Can you work these out from the model? Positions are in its coordinate system, mm. A direction names the side the tool comes from. Give positions to 0.01 mm unless a question says otherwise; leave off trailing zeros. Write each loop counter-clockwise with the first axis right and the second up, starting at its lowest first coordinate (ties: lowest second). Pieces come first, ordered by that corner, then holes.
1. I'm going to push flat-ended pins straight in: pin 1 (1.9 mm diameter, centred on x = -5.5, z = -10.5, fed in from -Y); pin 2 (1.5 mm diameter, centred on x = -5, z = -13, fed in from +Y); pin 3 (0.6 mm diameter, centred on x = 0.5, z = 0.5, fed in from -Y); pin 4 (1.5 mm diameter, centred on y = 0, z = -13.87, fed in from +X). Where does each tip first touch, or does it pass through?
2. Suppose I cut it at D-D (x = -3.75). Please give me the cut outline in (y, z), and give its area (3 significant figures).
3. If I drill on probe 1 along X at (y, z) = (-2.5, -7.25); probe 2 along Z at (x, y) = (-5.5, 0); probe 3 along Y at (x, z) = (-3.75, -13.75), over which ranges is the centre line in solid material (lowest first)?
4. Suppose I cut it at B-B (z = -8.25). Please give me the cut outline in (x, y), and give its area (3 significant figures).
5. On a 3-axis mill with a long thin cutter (end or side, diameter ignored), from which of +Z, -Z, +X, -X, +Y, -Y can I reach the whole of each face in a straight line? I mean faces 1 (the flat face through (-4, -4, -14.869)), 2 (the flat face through (-4, -5.002, -16)), 3 (the flat face through (1.25, 0, -10)). Say none if no direction works.
6. Thinking about a two-plate mould opening in Y: for faces 4 (the flat face through (4, -4, -14.869)), 5 (the cylindrical face through (-4.419, 0.577, -14.978)), 6 (the flat face through (0, -4, 0)), 7 (the flat face through (0, 4, 0)), which applies, pulls with the +Y half, pulls with the -Y half, needs draft (parallel to the pull), parting line crosses it, or undercut?
7. Suppose I cut it at A-A (y = 0). Please give me the cut outline in (x, z).
8. Suppose I cut it at C-C (z = -13.25). Please give me the cut outline in (x, y), and give its area (3 significant figures).
```python
from build123d import *

# Parameters (mm, degrees)
F0_R     = 1.25
F1_DEPTH = 7.5
F2_R     = 11
F3_DEPTH = 1.25


# Not quite as in the source:
# - a feature of the source that left no trace in its solid (it failed there, or was rolled back) is left out


with BuildPart() as f1:
    # F0 (on Right) → F1 (new body, symmetric)
    with BuildSketch(Plane.YZ):
        with BuildLine():
            Line((4, -1), (4, 1))
            Line((4, 1), (-4, 1))
            Line((-4, 1), (-4, -1))
            Line((-4, -1), (-3.4641016151, -1))
            ThreePointArc((-3.4641016151, -1), (-3.9803488917, -3.39600846), (-3.0021324352, -5.6433313908))
            Line((-3.0021324352, -5.6433313908), (-3.0021324352, -14.8694054575))
            Line((-3.0021324352, -14.8694054575), (-5.0021324352, -14.8694054575))
            Line((-5.0021324352, -14.8694054575), (-5.0021324352, -16.8694054575))
            Line((-5.0021324352, -16.8694054575), (3.9978675648, -16.8694054575))
            Line((3.9978675648, -16.8694054575), (3.9978675648, -14.8694054575))
            Line((3.9978675648, -14.8694054575), (3.9978675648, -3.1305945425))
            Line((3.9978675648, -3.1305945425), (3.9978675648, -2.8694054575))
            ThreePointArc((3.9978675648, -2.8694054575), (3.846285897, -1.901781079), (3.4641016151, -1))
            Line((3.4641016151, -1), (4, -1))
        make_face()
        with Locations((0, -13.8694054575)):
            Circle(F0_R, mode=Mode.SUBTRACT)
        with BuildLine():
            ThreePointArc((3.9978675648, -3.1305945425), (4, -3), (3.9978675648, -2.8694054575))
            Line((3.9978675648, -2.8694054575), (3.9978675648, -3.1305945425))
        make_face()
    extrude(amount=F1_DEPTH, both=True)

    # F2 (on Right) → F3 (cut, symmetric)
    with BuildSketch(Plane.YZ):
        with Locations((0, -13.8694054575)):
            Circle(F2_R)
    extrude(amount=F3_DEPTH, both=True, mode=Mode.SUBTRACT)


solid = f1.part
```
Checks:
1. pin 1: stops at y = -3
1. pin 2: stops at y = 4
1. pin 3: stops at y = -4
1. pin 4: passes through
2. outline: (-5, -16.87) - (4, -16.87) - (4, -3.13) arc R4 ccw to (3.46, -1) - (4, -1) - (4, 1) - (-4, 1) - (-4, -1) - (-3.46, -1) arc R4 ccw to (-3, -5.64) - (-3, -14.87) - (-5, -14.87) - close; hole circle Ø2.5 at (0, -13.87)
2. area: 129 mm2
3. probe 1: x = -7.5 to -1.25, 1.25 to 7.5
3. probe 2: z = -16.87 to -15.12, -12.62 to 1
3. probe 3: y = -3 to -1.24, 1.24 to 4
4. outline: (-7.5, -3) - (-1.25, -3) - (-1.25, 4) - (-7.5, 4) - close; (1.25, -3) - (7.5, -3) - (7.5, 4) - (1.25, 4) - close
4. area: 87.5 mm2
5. face 1: +X, -X, -Y
5. face 2: +Z, -Z, +X, -X, -Y
5. face 3: -Z
6. face 4: needs draft
6. face 5: undercut
6. face 6: pulls with the -Y half
6. face 7: pulls with the +Y half
7. outline: (-7.5, -16.87) - (-1.25, -16.87) - (-1.25, -15.12) - (-7.5, -15.12) - close; (-7.5, -12.62) - (-1.25, -12.62) - (-1.25, -2.87) - (1.25, -2.87) - (1.25, -12.62) - (7.5, -12.62) - (7.5, 1) - (-7.5, 1) - close; (1.25, -16.87) - (7.5, -16.87) - (7.5, -15.12) - (1.25, -15.12) - close
8. outline: (-7.5, -3) - (-1.25, -3) - (-1.25, -1.09) - (-7.5, -1.09) - close; (-7.5, 1.09) - (-1.25, 1.09) - (-1.25, 4) - (-7.5, 4) - close; (1.25, -3) - (7.5, -3) - (7.5, -1.09) - (1.25, -1.09) - close; (1.25, 1.09) - (7.5, 1.09) - (7.5, 4) - (1.25, 4) - close
8. area: 60.4 mm2
